Autodesk Inventor part; units mm, degrees
ref_plane "YZ Plane" through (0, 0, 0) normal (1, 0, 0) x (0, 1, 0)
ref_plane "XZ Plane" through (0, 0, 0) normal (0, 1, 0) x (-1, 0, 0)
ref_plane "XY Plane" through (0, 0, 0) normal (0, 0, 1) x (1, 0, 0)
sketch "Sketch1" plane through (0, 0, 0) normal (1, 0, 0) x (0, 1, 0)
  circle A0 centre (0, 0) radius 2.5
  dimension "d0" = 5
extrude "Extrusion1" add sketch "Sketch1" along normal blind 13
sketch "Sketch2" plane through (13, 0, 0) normal (1, 0, 0) x (0, 0, -1)
  circle A0 centre (0, 0) radius 3
  dimension "d3" = 6
extrude "Extrusion2" add sketch "Sketch2" along normal blind 53
chamfer "Chamfer1" distance 0.3 angle 45 2 edges at (0, -2.5, 0) (66, 0, 3)
thread "Thread1"
thread "Thread2"
properties part number "Piston Rod" material "Steel"
The model under review builds one solid part; all positions refer to its coordinate system, in mm. A direction names the side the tool comes from. Give positions to 0.01 mm unless a question says otherwise; leave off trailing zeros. Order: outer loops, then holes, each group sorted by start corner. A loop starts at its lowest first (then second) coordinate and runs counter-clockwise, first axis right, second up. Notation, with made-up numbers: (4.5, 66) -> (28.5, 66) arc R35 cw to (28.5, 103) -> close; hole circle Ø2 at (-24.5, 42.25). An arc over 180 degrees is marked (long way). Write item = value, one per line. Start each with the question number.
(1) For pin 1 Ø3 at (y, z) = (1, 1) entering from -X; pin 2 Ø1.5 at (x, y) = (38.5, -1.5) entering from +Z, all flat-tipped, find the tip position at first contact; note any pin that passes through.
(2) Take a section at A-A (y = 0). Write out the cut boundary in (x, z), plus the area to 3 significant figures.
(3) For L1, parallel to Y at x = 35, z = -1.65; L2, parallel to Y at x = 46, z = -0.6; L3, parallel to Z at x = 53, y = 1.05, list the stretches that pass through material, from the lowest coordinate up. Write a range as from..to.
(4) Take a section at D-D (x = 10.5). Write out the cut boundary in (y, z).
(5) Take a section at C-C (x = 57.5). Write out the cut boundary in (y, z), plus the area to 3 significant figures.
(6) Tool access review of faces 1 (the cylindrical face through (6.56, -0.54, 2.44)), 2 (the flat face through (66, 0, 0)): name each direction out of +Z, -Z, +X, -X, +Y, -Y from which nothing blocks a thin tool from reaching the whole face with its end or side.
Returned:
q1.pin_1 = 0
q1.pin_2 = 2.9
q2.outline = (0, -2.2) -> (0.3, -2.5) -> (13, -2.5) -> (13, -3) -> (65.7, -3) -> (66, -2.7) -> (66, 2.7) -> (65.7, 3) -> (13, 3) -> (13, 2.5) -> (0.3, 2.5) -> (0, 2.2) -> close
q2.area = 383 mm²
q3.L1 = -2.51..2.51
q3.L2 = -2.94..2.94
q3.L3 = -2.81..2.81
q4.outline = circle Ø5 at (0, 0)
q5.outline = circle Ø6 at (0, 0)
q5.area = 28.3 mm²
q6.face_1 = -X
q6.face_2 = +Z, -Z, +X, +Y, -Y
